Geometry: final body of the model. Coordinates: model frame, mm. A direction names the side the tool comes from. Coordinates: 2 decimals unless noted, no trailing zeros. Loops run counter-clockwise (first coordinate to the right, second up) from the corner with the lowest first, then second, coordinate; pieces in that order, holes last. Notation, with made-up numbers: M 21.25,89 L 25.25,89 A32 ccw 25.25,120 Z; hole C -20.5,-6 d10. An arc over 180 degrees is marked long. Write item = value, one per line. Start each with the question number.
```python
from build123d import *

# Parameters (mm, degrees)
SKETCH1_W           = 190.5
SKETCH1_H           = 25.4
BOSS_EXTRUDE1_DEPTH = 25.4
SKETCH2_W           = 9.525
SKETCH2_H           = 19.040717284
CUT_EXTRUDE1_DEPTH  = 508
SKETCH4_R           = 3.175
CUT_EXTRUDE3_DEPTH  = 508


with BuildPart() as part:
    # Sketch1 → Boss-Extrude1 (new body)
    with BuildSketch(Plane.XY):
        Rectangle(SKETCH1_W, SKETCH1_H)
    extrude(amount=BOSS_EXTRUDE1_DEPTH)

    # Sketch2 → Cut-Extrude1 (cut)
    with BuildSketch(Plane(origin=(95.25, 0, 0), x_dir=(0, 0, -1), z_dir=(1, 0, 0))):
        with Locations((-17.4625, 0)):
            Rectangle(SKETCH2_W, SKETCH2_H)
        with Locations((-7.9375, 0)):
            Rectangle(SKETCH2_W, SKETCH2_H)
    extrude(amount=-CUT_EXTRUDE1_DEPTH, mode=Mode.SUBTRACT)

    # Sketch4 → Cut-Extrude3 (cut)
    with BuildSketch(Plane.XY.offset(25.4)):
        with Locations((-82.55, 0)):
            Circle(SKETCH4_R)
        with Locations((82.55, 0)):
            Circle(SKETCH4_R)
    extrude(amount=-CUT_EXTRUDE3_DEPTH, mode=Mode.SUBTRACT)


solid = part.part
```
Item 1: Reachability of faces 4 (the flat face through (95.25, 11, 13)), 5 (the flat face through (1, 0, 22.225)) from +Z, -Z, +X, -X, +Y, -Y: full face, straight path, thin tool, end or side. Return the list, or none.
Item 2: Section query C-C (y = 6.75). Return the cut outline in (x, z) (3 decimals).
Item 3: First-contact query: pin 1 (5 mm diameter, centred on y = 9.5, z = 19, fed in from +X). Flat tip, straight axial feed; report the tip coordinate or a pass-through.
Item 4: Section query B-B (x = 82.55). Return the cut outline in (y, z) (3 decimals), plus the area to 3 significant figures.
Item 5: Pull-direction query (X, two-part tool) for faces 1 (the cylindrical face through (85.58, 0.95, 1.61)), 2 (the flat face through (-1, -12.7, 13)), 3 (the flat face through (-95.25, 11, 13)); classes: released by +X, released by -X, zero draft, split by the parting line, or undercut.
Item 6: Line query: line 1 (Z direction, x = -58, y = 2.5) (3 decimals); line 2 (Y direction, x = -10, z = 9). Output: solid intervals per line, ascending. Write a range as from..to.
Item 7: Section query D-D (x = -82). Return the cut outline in (y, z) (3 decimals), plus the area to 3 significant figures.
Item 8: Section query A-A (z = 11.5). Return the cut outline in (x, y), plus the area to 3 significant figures.
Verdict:
q1.face_4 = +Z, -Z, +X, +Y, -Y
q1.face_5 = +X, -X
q2.outline = M -95.25,0 L 95.25,0 L 95.25,3.175 L -95.25,3.175 Z; M -95.25,22.225 L 95.25,22.225 L 95.25,25.4 L -95.25,25.4 Z
q3.pin_1 = 95.25
q4.outline = M -12.7,0 L -3.175,0 L -3.175,3.175 L -9.52,3.175 L -9.52,22.225 L -3.175,22.225 L -3.175,25.4 L -12.7,25.4 Z; M 3.175,0 L 12.7,0 L 12.7,25.4 L 3.175,25.4 L 3.175,22.225 L 9.52,22.225 L 9.52,3.175 L 3.175,3.175 Z
q4.area = 242 mm2
q5.face_1 = undercut
q5.face_2 = zero draft
q5.face_3 = released by -X
q6.line_1 = 0..3.175, 22.225..25.4
q6.line_2 = -12.7..-9.52, 9.52..12.7
q7.outline = M -12.7,0 L -3.127,0 L -3.127,3.175 L -9.52,3.175 L -9.52,22.225 L -3.127,22.225 L -3.127,25.4 L -12.7,25.4 Z; M 3.127,0 L 12.7,0 L 12.7,25.4 L 3.127,25.4 L 3.127,22.225 L 9.52,22.225 L 9.52,3.175 L 3.127,3.175 Z
q7.area = 243 mm2
q8.outline = M -95.25,-12.7 L 95.25,-12.7 L 95.25,-9.52 L -95.25,-9.52 Z; M -95.25,9.52 L 95.25,9.52 L 95.25,12.7 L -95.25,12.7 Z
q8.area = 1,210 mm2
